Design review of the part built by this model. Coordinates are the model's own, in mm. Give positions to 0.01 mm unless a question says otherwise; leave off trailing zeros. Order: outer loops, then holes, each group sorted by start corner. A loop starts at its lowest first (then second) coordinate and runs counter-clockwise, first axis right, second up. Notation, with made-up numbers: M 69.25,30.25 L 109.25,30.25 A9 cw 109.25,41.25 Z; hole C 7.5,-38.75 d9. An arc over 180 degrees is marked long. Answer as a JSON object with one key per item and string values.
Autodesk Inventor part; units mm, degrees
ref_plane "YZ Plane" through (0, 0, 0) normal (1, 0, 0) x (0, 1, 0)
ref_plane "XZ Plane" through (0, 0, 0) normal (0, 1, 0) x (-1, 0, 0)
ref_plane "XY Plane" through (0, 0, 0) normal (0, 0, 1) x (1, 0, 0)
sketch "Sketch1" plane through (0, 0, 0) normal (0, 1, 0) x (-1, 0, 0)
  line L0 (0, 0) -> (40, 0)
  line L1 (40, 0) -> (40, -25)
  line L2 (40, -25) -> (0, -25)
  line L3 (0, -25) -> (0, 0)
  circle A0 centre (37, -3) radius 1
  line L4 (40, -12.5) -> (0, -12.5)
  line L5 (20, 0) -> (20, -25)
  circle A1 centre (37, -22) radius 1
  circle A2 centre (3, -3) radius 1
  circle A3 centre (3, -22) radius 1
  dimension "d0" = 40
  dimension "d1" = 25
  dimension "d2" = 2
  dimension "d3" = 3
  dimension "d4" = 3
extrude "Extrusion1" add sketch "Sketch1" along normal blind 3
fillet "Fillet1" radius 2 4 edges at (0, 1.5, 0) (0, 1.5, -25) (-40, 1.5, -25) (-40, 1.5, 0)
properties part number "SpojovaciDeska"
(1) We need section B-B (x = -3). Write out the cut boundary in (y, z), plus the area to 3 significant figures.
Checked values:
{"outline": "M 0,-25 L 3,-25 L 3,-23 L 0,-23 Z; M 0,-21 L 3,-21 L 3,-4 L 0,-4 Z; M 0,-2 L 3,-2 L 3,0 L 0,0 Z", "area": "63.0 mm^2"}
(2) To check wall thickness, follow L1, parallel to Z at x = -37, y = 2; L2, parallel to X at y = 2.35, z = -22.25; L3, parallel to X at y = 1.95, z = -23.5. State the ranges of each line that lie inside material, in increasing order. Write a range as from..to.
Checked values:
{"L1": "z = -25..-23, -21..-4, -2..0", "L2": "x = -40..-37.97, -36.03..-3.97, -2.03..0", "L3": "x = -39.94..-0.06"}
(3) We need section C-C (y = 2.5). Write out the cut boundary in (x, z).
Checked values:
{"outline": "M -40,-23 A2 ccw -38,-25 L -2,-25 A2 ccw 0,-23 L 0,-2 A2 ccw -2,0 L -38,0 A2 ccw -40,-2 Z; hole C -37,-22 d2; hole C -37,-3 d2; hole C -3,-22 d2; hole C -3,-3 d2"}
(4) Draft analysis for pull direction Z (two halves, no side actions). For faces 1 (the flat face through (-20, 1, -25)), 2 (the cylindrical face through (-37, 1, -21)), 3 (the flat face through (-20, 3, -12)), state which applies: +Z half, -Z half, draft (parallel to the pull), parting line (faces both ways), or undercut.
Checked values:
{"face 1": "-Z half", "face 2": "undercut", "face 3": "draft"}
(5) We need section A-A (z = -3). Write out the cut boundary in (x, y), plus the area to 3 significant figures.
Checked values:
{"outline": "M -40,0 L -38,0 L -38,3 L -40,3 Z; M -36,0 L -4,0 L -4,3 L -36,3 Z; M -2,0 L 0,0 L 0,3 L -2,3 Z", "area": "108 mm^2"}
